Verification items for the finished model (mm, model axes). A direction names the side the tool comes from. Round coordinates to 2 decimals unless told otherwise and drop trailing zeros. Order: outer loops, then holes, each group sorted by start corner. A loop starts at its lowest first (then second) coordinate and runs counter-clockwise, first axis right, second up. Notation, with made-up numbers: M 14.5,41.25 L 23.5,41.25 A26 ccw 23.5,70.25 Z; hole C 13.5,40.25 d9. An arc over 180 degrees is marked long. Use CSV: the item, a comma, the result in double quotes. Start each with the question number.
Q1. Set-up check for faces 4 (the face through (94.297, 5.07, 6.014)), 5 (the face through (-38.93, 2.83, 19.72)), 6 (the face through (68, 10, 20)): record each of +Z, -Z, +X, -X, +Y, -Y from which the full face is reachable in a straight line by a thin tool's end or side.
Q2. Sectioned sample at D-D (z = 25.5). Enter the section's corners in (x, y), and give its area (3 significant figures).
Q3. Gauge pin test, flat ends, axial feed: pin 1 Ø17 at (x, z) = (80, 20) entering from +Y; pin 2 Ø13.5 at (x, z) = (-80, 20) entering from -Y. Record the tip position at first contact, or that the pin passes through.
Q4. Scan lines: line 1 (X direction, y = 7.5, z = 20); line 2 (X direction, y = 6, z = 20); line 3 (Y direction, x = -83.5, z = 34). Record each from-to range of solid material in increasing order.
Q5. Mould release check, pull along X, two halves, no side actions. Record for faces 1 (the face through (-68, 10, 20)), 2 (the face through (38.7, 3, 19.7)), 3 (the face through (0.798, 44.993, 19.72)): +X half, -X half, draft (parallel to the pull), parting line (faces both ways), or undercut.
Q6. Sectioned sample at A-A (y = 31.5). Enter the section's corners in (x, z), and give its area (3 significant figures).
Q7. Sectioned sample at B-B (z = 17). Enter the section's corners in (x, y), and give its area (3 significant figures).
Q8. Sectioned sample at C-C (x = 54). Enter the section's corners in (y, z), and give its area (3 significant figures).
```python
from build123d import *

# Parameters (mm, degrees)
BOSS_EXTRUDE1_DEPTH = 40
FILLET1_R           = 20
SKETCH2_R           = 7.5
CUT_EXTRUDE1_DEPTH  = 114.247516529


with BuildPart() as part:
    # Sketch1 → Boss-Extrude1 (new body)
    with BuildSketch(Plane.XY):
        with BuildLine():
            Line((-100, 0), (-47.696960071, 0))
            ThreePointArc((-47.696960071, 0), (-38.822840396, 2.906613378), (-33.38787205, 10.5))
            ThreePointArc((-33.38787205, 10.5), (0, 35), (33.38787205, 10.5))
            ThreePointArc((33.38787205, 10.5), (38.822840396, 2.906613378), (47.696960071, 0))
            Line((47.696960071, 0), (100, 0))
            Line((100, 0), (100, 10))
            Line((100, 10), (47.696960071, 10))
            ThreePointArc((47.696960071, 10), (44.738920179, 10.968871126), (42.927264064, 13.5))
            ThreePointArc((42.927264064, 13.5), (0, 45), (-42.927264064, 13.5))
            ThreePointArc((-42.927264064, 13.5), (-44.738920179, 10.968871126), (-47.696960071, 10))
            Line((-47.696960071, 10), (-100, 10))
            Line((-100, 10), (-100, 0))
        make_face()
    extrude(amount=BOSS_EXTRUDE1_DEPTH)

    # Fillet1
    fillet1_edges = [part.edges().sort_by_distance(p)[0] for p in [
        (100, 5, 0),
        (100, 5, 40),
        (-100, 5, 0),
        (-100, 5, 40),
    ]]
    fillet(fillet1_edges, radius=FILLET1_R - 0.0001)  # a hair under: the kernel refuses the full size

    # Sketch2 → Cut-Extrude1 (cut, through all)
    with BuildSketch(Plane(origin=(0, 10, 0), x_dir=(1, 0, 0), z_dir=(0, 1, 0))):
        with Locations(Location((-80, -20, 0), (0, 0, 270))):
            Circle(SKETCH2_R)
        with Locations(Location((80, -20, 0), (0, 0, 270))):
            Circle(SKETCH2_R)
    extrude(amount=-CUT_EXTRUDE1_DEPTH, mode=Mode.SUBTRACT)


solid = part.part
```
Verdict:
1,face 4,"-Z, +X, +Y, -Y"
1,face 5,"+Z, -Z, -Y"
1,face 6,"+Z, -Z, +X, +Y"
2,outline,"M -99.23,0 L -85.1,0 L -85.1,10 L -99.23,10 Z; M -74.9,0 L -47.7,0 A15 ccw -33.39,10.5 A35 cw 33.39,10.5 A15 ccw 47.7,0 L 74.9,0 L 74.9,10 L 47.7,10 A5 cw 42.93,13.5 A45 ccw -42.93,13.5 A5 cw -47.7,10 L -74.9,10 Z; M 85.1,0 L 99.23,0 L 99.23,10 L 85.1,10 Z"
2,area,"2,090 mm²"
3,pin 1,"stops at y = 10"
3,pin 2,"passes through"
4,line 1,"x = -100 to -87.5, -72.5 to -34.71, 34.71 to 72.5, 87.5 to 100"
4,line 2,"x = -100 to -87.5, -72.5 to -35.7, 35.7 to 72.5, 87.5 to 100"
4,line 3,"y = 0 to 10"
5,face 1,"draft"
5,face 2,"undercut"
5,face 3,"parting line"
6,outline,"M -32.14,0 L -15.26,0 L -15.26,40 L -32.14,40 Z; M 15.26,0 L 32.14,0 L 32.14,40 L 15.26,40 Z"
6,area,"1,350 mm²"
7,outline,"M -99.77,0 L -86.87,0 L -86.87,10 L -99.77,10 Z; M -73.13,0 L -47.7,0 A15 ccw -33.39,10.5 A35 cw 33.39,10.5 A15 ccw 47.7,0 L 73.13,0 L 73.13,10 L 47.7,10 A5 cw 42.93,13.5 A45 ccw -42.93,13.5 A5 cw -47.7,10 L -73.13,10 Z; M 86.87,0 L 99.77,0 L 99.77,10 L 86.87,10 Z"
7,area,"2,030 mm²"
8,outline,"M 0,0 L 10,0 L 10,40 L 0,40 Z"
8,area,"400 mm²"
